Geometry check sheet. Reference: the model listing, model coordinates, mm. A direction names the side the tool comes from. Round coordinates to 2 decimals unless told otherwise and drop trailing zeros. Write each loop counter-clockwise with the first axis right and the second up, starting at its lowest first coordinate (ties: lowest second). Pieces come first, ordered by that corner, then holes.
from build123d import *

# Parameters (mm, degrees)
F0_R      = 4.75
F1_DEPTH  = 7.5
F2_R      = 2.125
F3_DEPTH  = 25
F4_R      = 7.825
F5_DEPTH  = 5
F6_SIZE   = 2.5
F8_DEPTH  = 19.5
F9_R      = 2.125
F10_DEPTH = 25


# Not quite as in the source:
# - a pattern or mirror of a feature is missing from the dataset's text; its kind, count and spacing are read off the source's solid


with BuildPart() as f1:
    # F0 (on Top) → F1 (new body, symmetric)
    with BuildSketch(Plane.XY):
        with BuildLine():
            Line((-25.9795548635, -11.025), (0, -11.025))
            Line((0, -11.025), (25.9795548635, -11.025))
            Line((25.9795548635, -11.025), (25.9795548635, -6.025))
            Line((25.9795548635, -6.025), (10.9795548635, -6.025))
            Line((10.9795548635, -6.025), (10.9795548635, 1))
            ThreePointArc((10.9795548635, 1), (7.4338961857, 8.1417327701), (0, 11.025))
            ThreePointArc((0, 11.025), (-7.4338961857, 8.1417327701), (-10.9795548635, 1))
            Line((-10.9795548635, 1), (-10.9795548635, -6.025))
            Line((-10.9795548635, -6.025), (-25.9795548635, -6.025))
            Line((-25.9795548635, -6.025), (-25.9795548635, -11.025))
        make_face()
        Circle(F0_R, mode=Mode.SUBTRACT)
    extrude(amount=F1_DEPTH, both=True)

    # F2 (on face) → F3 (cut)
    with BuildSketch(Plane.XZ.offset(11.025)):
        with Locations((-18.4795548635, 0)):
            Circle(F2_R)
        with Locations((18.4795548635, 0)):
            Circle(F2_R)
    extrude(amount=-F3_DEPTH, mode=Mode.SUBTRACT)

    # F4 (on face) → F5 (cut)
    with BuildSketch(Plane.XY.offset(7.5)):
        Circle(F4_R)
    f5 = extrude(amount=-F5_DEPTH, mode=Mode.SUBTRACT)

    # F5_copies: F5 across plane
    add(f5.mirror(Plane(origin=(0, 0, 0), x_dir=(-1, 0, 0), z_dir=(0, 0, -1))), mode=Mode.SUBTRACT)

    # F6
    f6_edges = [f1.edges().sort_by_distance(p)[0] for p in [
        (-10.979555, -6.025, 0),
        (10.979555, -6.025, 0),
    ]]
    chamfer(f6_edges, length=F6_SIZE)

    # F7 (on face) → F8 (join)
    with BuildSketch(Plane.XY.offset(7.5)):
        with BuildLine():
            Line((-25.9795548635, -11.025), (0, -11.025))
            Line((0, -11.025), (25.9795548635, -11.025))
            Line((25.9795548635, -11.025), (25.9795548635, -6.025))
            Line((25.9795548635, -6.025), (10.9795548635, -6.025))
            Line((10.9795548635, -6.025), (10.9795548635, 0))
            Line((10.9795548635, 0), (7.825, 0))
            ThreePointArc((7.825, 0), (0, -7.825), (-7.825, 0))
            Line((-7.825, 0), (-10.9795548635, 0))
            Line((-10.9795548635, 0), (-10.9795548635, -6.025))
            Line((-10.9795548635, -6.025), (-25.9795548635, -6.025))
            Line((-25.9795548635, -6.025), (-25.9795548635, -11.025))
        make_face()
    f8 = extrude(amount=F8_DEPTH)

    # F8_copies: F8 across plane
    add(f8.mirror(Plane(origin=(0, 0, 0), x_dir=(-1, 0, 0), z_dir=(0, 0, -1))))

    # F9 (on face) → F10 (cut)
    with BuildSketch(Plane(origin=(0, -6.025, 0), x_dir=(-1, 0, 0), z_dir=(0, 1, 0))):
        with Locations((-18.4795548635, 19.5)):
            Circle(F9_R)
        with Locations((18.4795548635, 19.5)):
            Circle(F9_R)
    f10 = extrude(amount=-F10_DEPTH, mode=Mode.SUBTRACT)

    # F10_copies: F10 across plane
    add(f10.mirror(Plane(origin=(0, 0, 0), x_dir=(-1, 0, 0), z_dir=(0, 0, -1))), mode=Mode.SUBTRACT)


solid = f1.part
1. Section check D-D (z = 14). Record the cut outline in (x, y) (3 decimals).
2. Scan lines: line 1 along X through (y, z) = (-7.2, -19.5); line 2 along X through (y, z) = (-0.25, 16); line 3 along X through (y, z) = (-7, -19.5). Record each from-to range of solid material in increasing order.
3. Section check B-B (y = -1.75). Record the cut outline in (x, z), plus the area to 3 significant figures.
4. Section check A-A (z = 0). Record the cut outline in (x, y) (3 decimals).
5. Release check for a two-part mould opening along Z. For faces 4 (the face through (0, -5, -2.5)), 5 (the face through (-1.02, -7.76, 11.86)), 6 (the face through (-19.622, -8.49, 21.292)), 7 (the face through (12, -5, 7.5)) record: +Z half, -Z half, draft (parallel to the pull), parting line (faces both ways), or undercut.
6. Depth check by flat-ended pin: pin 1 Ø0.9 at (x, z) = (9, 22) entering from +Y; pin 2 Ø1.3 at (x, y) = (12.5, -4.5) entering from +Z; pin 3 Ø6 at (x, y) = (-3.5, -3) entering from -Z; pin 4 Ø2.5 at (x, z) = (18.48, 0) entering from -Y. Enter the tip coordinate at first touch or a pass-through.
7. Access from +Z, -Z, +X, -X, +Y, -Y to the whole of each face (thin tool, end or side, straight path). Record for faces 1 (the face through (-9, 0, 17)), 2 (the face through (0, -5, 2.5)), 3 (the face through (9, 0, -17)).
8. Section check C-C (z = 20.5). Record the cut outline in (x, y) (3 decimals).
Results below:
1. outline: (-25.98, -11.025) - (25.98, -11.025) - (25.98, -6.025) - (10.98, -6.025) - (10.98, 0) - (7.825, 0) arc R7.825 cw to (-7.825, 0) - (-10.98, 0) - (-10.98, -6.025) - (-25.98, -6.025) - close
2. line 1: x = -25.98 to -20.6, -16.35 to -3.06, 3.06 to 16.35, 20.6 to 25.98
2. line 2: x = -10.98 to -7.82, 7.82 to 10.98
2. line 3: x = -25.98 to -20.6, -16.35 to -3.5, 3.5 to 16.35, 20.6 to 25.98
3. outline: (-10.98, -27) - (-7.63, -27) - (-7.63, -2.5) - (-4.42, -2.5) - (-4.42, 2.5) - (-7.63, 2.5) - (-7.63, 27) - (-10.98, 27) - close; (4.42, -2.5) - (7.63, -2.5) - (7.63, -27) - (10.98, -27) - (10.98, 27) - (7.63, 27) - (7.63, 2.5) - (4.42, 2.5) - close
3. area: 394 mm2
4. outline: (-25.98, -11.025) - (-20.605, -11.025) - (-20.605, -6.025) - (-25.98, -6.025) - close; (-16.355, -11.025) - (16.355, -11.025) - (16.355, -6.025) - (13.48, -6.025) - (10.98, -3.525) - (10.98, 1) arc R11.025 ccw to (-10.98, 1) - (-10.98, -3.525) - (-13.48, -6.025) - (-16.355, -6.025) - close; (20.605, -11.025) - (25.98, -11.025) - (25.98, -6.025) - (20.605, -6.025) - close; hole circle Ø9.5 at (0, 0)
5. face 4: -Z half
5. face 5: draft
5. face 6: undercut
5. face 7: +Z half
6. pin 1: stops at y = 0
6. pin 2: stops at z = 7.5
6. pin 3: stops at z = -2.5
6. pin 4: passes through
7. face 1: +Z, +X, -X, +Y
7. face 2: +Z
7. face 3: -Z, +X, -X, +Y
8. outline: (-25.98, -11.025) - (-20.355, -11.025) - (-20.355, -6.025) - (-25.98, -6.025) - close; (-16.605, -11.025) - (16.605, -11.025) - (16.605, -6.025) - (10.98, -6.025) - (10.98, 0) - (7.825, 0) arc R7.825 cw to (-7.825, 0) - (-10.98, 0) - (-10.98, -6.025) - (-16.605, -6.025) - close; (20.355, -11.025) - (25.98, -11.025) - (25.98, -6.025) - (20.355, -6.025) - close
